```python
from build123d import *

# Parameters (mm, degrees)
F2_W     = 15
F2_H     = 7
F2_R     = 1.5
F3_DEPTH = 2.000000095
F4_R     = 1
F5_SIZE  = 0.99999


# Not quite as in the source:
# - a fillet or chamfer is up to 0.001 mm smaller than in the source, because OpenCascade refuses the exact size


with BuildPart() as f1:
    # F0 (on Front) → F1 (revolve)
    with BuildSketch(Plane.XZ):
        with BuildLine():
            Line((-1.5, 4), (-1.5, 0))
            Line((-1.5, 0), (0, 0))
            Line((0, 0), (0, 9.5980762114))
            ThreePointArc((0, 9.5980762114), (-2.8977774789, 7.3745333467), (-1.5, 4))
        make_face()
    revolve(axis=Axis((0, 0, 4.7990381057), (0, 0, 1)))

    # F2 (on face) → F3 (join)
    with BuildSketch(Plane(origin=(0, 0, 0), x_dir=(1, 0, 0), z_dir=(0, 0, -1))):
        Rectangle(F2_W, F2_H)
        Circle(F2_R, mode=Mode.SUBTRACT)
        Circle(F2_R)
    extrude(amount=F3_DEPTH)

    # F4
    f4_edges = [f1.edges().sort_by_distance(p)[0] for p in [
        (1.5, 0, 0),
        (1.5, 0, 4),
    ]]
    fillet(f4_edges, radius=F4_R)

    # F5 (size 1 in the source; OpenCascade refuses exactly that, so slightly less here)
    f5_edges = [f1.edges().sort_by_distance(p)[0] for p in [
        (2.5, 0, 0),
        (7.5, 0, 0),
        (0, 3.5, 0),
        (0, -3.5, 0),
        (-7.5, 0, 0),
    ]]
    chamfer(f5_edges, length=F5_SIZE)


solid = f1.part
```
Source: CAD feature listing. Evaluate the final solid. Frame: model axes, mm. Round coordinates to 2 decimals unless told otherwise and drop trailing zeros. Loops run counter-clockwise (first coordinate to the right, second up) from the corner with the lowest first, then second, coordinate; pieces in that order, holes last. Notation, with made-up numbers: M -15.5,86 L 2.5,86 A21 cw 2.5,98 Z; hole C 28,83.5 d7. An arc over 180 degrees is marked long. Put each result on its own line as item: value.
(1) Section B-B, the plane y = 2.75. Return loops of the section in (x, z).
Solutions:
outline: M -7.5,-2 L 7.5,-2 L 7.5,-1 L 6.75,-0.25 L -6.75,-0.25 L -7.5,-1 Z; C 0,6.6 d2.4
(2) Pull-direction query (Z, two-part tool) for faces 1 (the face through (7, 0, -0.5)), 2 (the face through (0.195, -1.487, 2.22)), 3 (the face through (-0.1, 3.5, -1.5)), 4 (the face through (0, 0, -2)); classes: released by +Z, released by -Z, zero draft, split by the parting line, or undercut.
Solutions:
face 1: released by +Z
face 2: undercut
face 3: zero draft
face 4: released by -Z
(3) Section C-C, the plane z = 4.5. Return loops of the section in (x, y).
Solutions:
outline: C 0,0 d4.29
(4) Ray query, line 1 (Z direction, x = -6, y = 0.75); line 2 (Y direction, x = 6.5, z = -0.5); line 3 (X direction, y = 1, z = 3.25). Return the intervals inside material, ascending. Write a range as [from, to].
Solutions:
line 1: [-2, 0]
line 2: [-3, 3]
line 3: [-1.12, 1.12]
(5) First-contact query: pin 1 (4 mm diameter, centred on x = -2.5, y = 0.5, fed in from +Z); pin 2 (1 mm diameter, centred on y = -2.5, z = 7.5, fed in from +X); pin 3 (4 mm diameter, centred on y = -1, z = 3.5, fed in from +X). Flat tips, straight axial feed; report the tip coordinate or a pass-through.
Solutions:
pin 1: z = 9.55
pin 2: x = 2.08
pin 3: x = 2.72
(6) Section A-A, the plane x = 5.5. Return loops of the section in (y, z), and give its area (3 significant figures).
Solutions:
outline: M -3.5,-2 L 3.5,-2 L 3.5,-1 L 2.5,0 L -2.5,0 L -3.5,-1 Z
area: 13.0 mm²
